Can you work these out from the model? Positions are in its coordinate system, mm. Face numbers are marked on the shaded views. A direction names the side the tool comes from. Coordinates: 2 decimals unless noted, no trailing zeros. Order: outer loops, then holes, each group sorted by start corner. A loop starts at its lowest first (then second) coordinate and runs counter-clockwise, first axis right, second up. Notation, with made-up numbers: (79, 61) -> (136, 61) arc R28 cw to (136, 86) -> close; hole circle Ø9 at (-15.5, 14.25). An arc over 180 degrees is marked (long way). Answer as CSV lines item,"result".
from build123d import *

# Parameters (mm, degrees)
SKETCH1_R                    = 20
EXTRUDE1_DEPTH               = 12.5
SKETCH2_W                    = 25
SKETCH2_H                    = 400
EXTRUDE2_DEPTH               = 100
FILLET1_R                    = 40
F_5_8_0_625_DIAMETER_HOLE1_D = 15.875
CHAMFER1_SIZE                = 100
FILLET2_R                    = 10


with BuildPart() as part:
    # Sketch1 → Extrude1 (new, symmetric)
    with BuildSketch(Plane(origin=(0, 0, 0), x_dir=(0, 0, -1), z_dir=(1, 0, 0))):
        with BuildLine():
            Line((0, 50), (-550, 50))
            Line((-550, 50), (-550, -350))
            Line((-550, -350), (-400, -350))
            Line((-400, -350), (-400, -50))
            Line((-400, -50), (0, -50))
            ThreePointArc((0, -50), (50, 0), (0, 50))
        make_face()
        Circle(SKETCH1_R, mode=Mode.SUBTRACT)
        with Locations((-425, -70)):
            Circle(SKETCH1_R, mode=Mode.SUBTRACT)
    extrude(amount=EXTRUDE1_DEPTH, both=True)

    # Sketch2 → Extrude2 (add)
    with BuildSketch(Plane(origin=(12.5, 0, 0), x_dir=(0, 0, -1), z_dir=(1, 0, 0))):
        with Locations((-537.5, -150)):
            Rectangle(SKETCH2_W, SKETCH2_H)
    extrude(amount=EXTRUDE2_DEPTH)

    # Fillet1
    fillet1_edges = [part.edges().sort_by_distance(p)[0] for p in [
        (112.5, -350, 537.5),
        (112.5, 50, 537.5),
        (0, -350, 400),
    ]]
    fillet(fillet1_edges, radius=FILLET1_R)

    # 5/8 (0.625) Diameter Hole1 (through all)
    with Locations(Plane.XY.offset(550)):
        with Locations((72.5, 10), (72.5, -310)):
            Hole(F_5_8_0_625_DIAMETER_HOLE1_D / 2)

    # Chamfer1
    chamfer1_edges = [part.edges().sort_by_distance(p)[0] for p in [
        (0, -50, 400),
    ]]
    chamfer(chamfer1_edges, length=CHAMFER1_SIZE)

    # Fillet2
    fillet2_edges = [part.edges().sort_by_distance(p)[0] for p in [
        (12.5, -150, 525),
        (-12.5, -150, 550),
    ]]
    fillet(fillet2_edges, radius=FILLET2_R)


solid = part.part
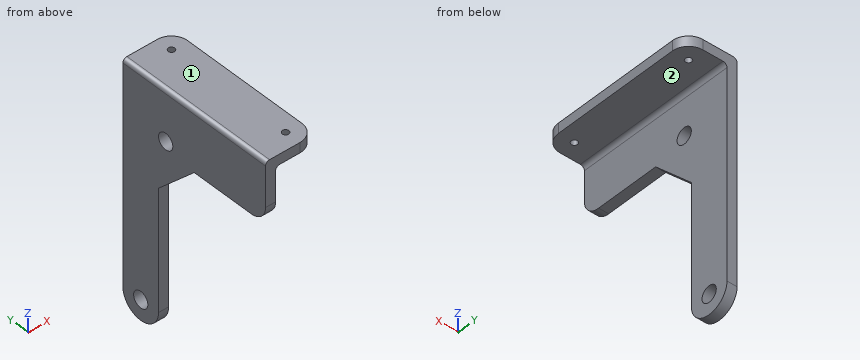
Q1. For P1, Ø20, axis at x = -1, z = 157, coming from the -Y side; P2, Ø18.5, axis at x = 72.5, y = -310, coming from the +Z side; P3, Ø7.5, axis at x = 1.5, y = -256.5, coming from the -Z side; P4, Ø12, axis at x = 90, y = -209.5, coming from the -Z side, each with a flat end and sliding along its axis, tell me the tip position at first contact or that it passes through.
Solution:
P1,"y = -50"
P2,"z = 550"
P3,"z = 400"
P4,"z = 525"
Q2. Imagine slicing it at D-D (z = 272.5). List the corners of the cut face in (x, y) for me.
Solution:
outline,"(-12.5, -50) -> (12.5, -50) -> (12.5, 50) -> (-12.5, 50) -> close"
Q3. Imagine slicing it at C-C (x = 50). List the corners of the cut face in (y, z) for me.
Solution:
outline,"(-350, 525) -> (50, 525) -> (50, 550) -> (-350, 550) -> close"
Q4. Which directions (+Z, -Z, +X, -X, +Y, -Y) give clear straight access to the entire face, cutting with the end or side of a thin tool? Please do the marked faces 1 and 2.
Solution:
face 1,"+Z, +X, -X, +Y, -Y"
face 2,"-Z, +X, +Y, -Y"
Q5. If I drill on line 1 (Y direction, x = 72.5, z = 533.5); line 2 (Y direction, x = 0, z = 0); line 3 (Z direction, x = 75, y = 20), over which ranges is the centre line in solid material (lowest first)?
Solution:
line 1,"-350 to -317.94, -302.06 to 2.06, 17.94 to 50"
line 2,"-50 to -20, 20 to 50"
line 3,"525 to 550"
Q6. Imagine slicing it at B-B (y = -120). List the corners of the cut face in (x, z) for me, and give its area (3 significant figures).
Solution:
outline,"(-12.5, 370) -> (12.5, 370) -> (12.5, 515) arc R10 cw to (22.5, 525) -> (112.5, 525) -> (112.5, 550) -> (-2.5, 550) arc R10 ccw to (-12.5, 540) -> close"
area,"7,000 mm2"
Q7. Imagine slicing it at A-A (y = -70). List the corners of the cut face in (x, z) for me.
Solution:
outline,"(-12.5, 320) -> (12.5, 320) -> (12.5, 405) -> (-12.5, 405) -> close; (-12.5, 445) -> (12.5, 445) -> (12.5, 515) arc R10 cw to (22.5, 525) -> (112.5, 525) -> (112.5, 550) -> (-2.5, 550) arc R10 ccw to (-12.5, 540) -> close"
